Here's how the part is built. I have some questions about the finished solid (model axes, mm). Face numbers are marked on the shaded views. Round coordinates to 2 decimals unless told otherwise and drop trailing zeros. Write each loop counter-clockwise with the first axis right and the second up, starting at its lowest first coordinate (ties: lowest second). Pieces come first, ordered by that corner, then holes. Notation, with made-up numbers: (7, 51.25) -> (46, 51.25) arc R3 ccw to (46, 55.25) -> close; hole circle Ø2 at (79.25, 66.5). An arc over 180 degrees is marked (long way). Put each result on its own line as item: value. Start each with the question number.
1) Will these pins go through, and if not, where does the flat tip stop? P1, Ø8, axis at x = -32.5, z = 18.5, coming from the +Y side; P2, Ø6, axis at x = 0, z = 12.5, coming from the +Y side; P3, Ø6, axis at y = 42.5, z = 18.5, coming from the -X side.
2) We'd pull the mould along Y, two halves only. Please class the marked faces 1, 2 and 3: released by +Y, released by -Y, zero draft, split by the parting line, or undercut.
3) If I drill on line 1 along Z through (x, y) = (-1.5, -45); line 2 along X through (y, z) = (-11.5, 21); line 3 along Y through (x, z) = (-22.5, 7), over which ranges is the centre line in solid material (lowest first)? Write a range as [from, to].
4) I want a section at B-B, the plane z = 17.5. List the corners of the cut face in (x, y) for me, then the cut area to 3 significant figures.
5) I want a section at A-A, the plane z = 9. List the corners of the cut face in (x, y) for me.
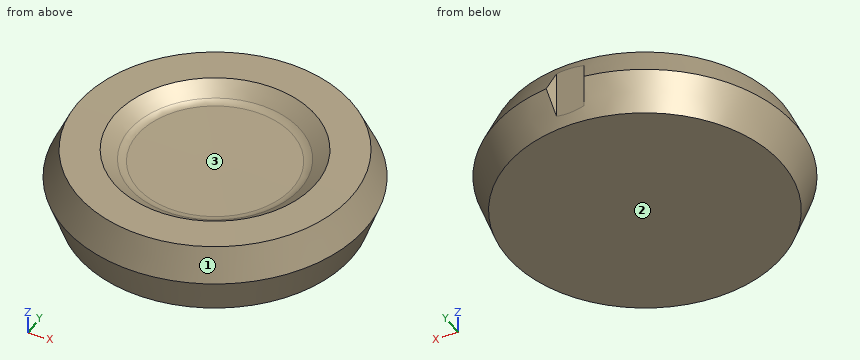
from build123d import *

# Parameters (mm, degrees)
F2_R     = 5
F5_DEPTH = 25


with BuildPart() as f1:
    # F0 (on Front) → F1 (revolve)
    with BuildSketch(Plane.XZ):
        Polygon((-29.923142, 20.133244), (-36.73585, 24.941483), (-49.877202, 25), (-55, 13.824025), (-50, 0), (0, 0), (0, 20), align=None)
    revolve(axis=Axis((0, 0, 10), (0, 0, -1)))

    # F2
    f2_edges = [f1.edges().sort_by_distance(p)[0] for p in [
        (29.923142, 0, 20.133244),
    ]]
    fillet(f2_edges, radius=F2_R)

    # F4 (on offset) → F5 (cut)
    with BuildSketch(Plane.XY.offset(25)):
        Polygon((9.998686, 59.837915), (5.139713, 68.578074), (-4.858973, 68.740159), (-9.998686, 60.162085), (-5.139713, 51.421926), (4.858973, 51.259841), align=None)
    extrude(amount=-F5_DEPTH, mode=Mode.SUBTRACT)


solid = f1.part
Findings:
1. P1: stops at y = 45.31
1. P2: stops at y = 51.39
1. P3: stops at x = -35.71
2. face 1: split by the parting line
2. face 2: zero draft
2. face 3: undercut
3. line 1: z = [0, 24.98]
3. line 2: x = [-50.42, -28.95], [28.95, 50.42]
3. line 3: y = [-47.47, 47.47]
4. outline: (-6, 52.98) arc R53.32 ccw (long way) to (5.89, 52.99) -> (4.86, 51.26) -> (-5.14, 51.42) -> close
4. area: 8,910 mm2
5. outline: (-5.97, 52.92) arc R53.26 ccw (long way) to (5.86, 52.93) -> (4.86, 51.26) -> (-5.14, 51.42) -> close
